Read the model definition and answer for the solid it produces. Units are mm, in the model's axes. A direction names the side the tool comes from. Give positions to 0.01 mm unless a question says otherwise; leave off trailing zeros. Loops run counter-clockwise (first coordinate to the right, second up) from the corner with the lowest first, then second, coordinate; pieces in that order, holes last. Notation, with made-up numbers: (-23.75, 59) -> (30.25, 59) arc R27 ccw to (30.25, 93) -> close; hole circle Ø3 at (70.25, 9). An arc over 180 degrees is marked (long way). Write each question's results on one line, items separated by ' | '. Start each with the question number.
Item 1: Section C-C on y = 6.25 is taken. State how many separate pieces and enclosed holes the cut face has, and give its area (3 significant figures).
Item 2: Section B-B on z = -1.5 is taken. Write down the section's boundary in (x, y).
Item 3: Find the intervals of material crossed by line 1 (Z direction, x = 0, y = 20.25); line 2 (Z direction, x = 0, y = 15.5); line 3 (Z direction, x = 2.25, y = 6.5), in increasing order.
Item 4: Determine the mould class of faces 1 (the flat face through (-2.6, 25.4, 0.2)), 2 (the flat face through (0, 20.32, 0)), 3 (the flat face through (-0.44, 22.9, -1.78)), 4 (the flat face through (3, 13, 12.7)) for opening direction Z: +Z half, -Z half, draft (parallel to the pull), parting line (faces both ways), or undercut.
Item 5: Which of the six approach directions +Z, -Z, +X, -X, +Y, -Y give full straight-line access (tool end or side, diameter ignored) to faces 5 (the flat face through (-4, 23, -0.177)), 6 (the cylindrical face through (-0.69, 12.88, -4.84))?
Item 6: Section A-A on z = -6.75 is taken. Write down the section's boundary in (x, y).
Autodesk Inventor part; units mm, degrees
ref_plane "YZ Plane" through (0, 0, 0) normal (1, 0, 0) x (0, 1, 0)
ref_plane "XZ Plane" through (0, 0, 0) normal (0, 1, 0) x (-1, 0, 0)
ref_plane "XY Plane" through (0, 0, 0) normal (0, 0, 1) x (1, 0, 0)
sketch "Sketch1" plane through (0, 0, 0) normal (0, 1, 0) x (-1, 0, 0)
  line L0 (12.7, 12.7) -> (-12.7, 12.7)
  line L1 (-12.7, 12.7) -> (-12.7, -12.7)
  line L2 (-12.7, -12.7) -> (12.7, -12.7)
  line L3 (12.7, -12.7) -> (12.7, 12.7)
  line L4 (12.7, 12.7) -> (-12.7, -12.7) construction
  line L5 (-12.7, 12.7) -> (12.7, -12.7) construction
  point P0 (0, 0)
  dimension "d0" = 25.4
  dimension "d1" = 25.4
extrude "Extrusion1" add sketch "Sketch1" along normal blind 25.4
sketch "Sketch2" plane through (0, 25.4, 0) normal (0, 1, 0) x (1, 0, 0)
  line L0 (-12.7, 12.7) -> (-12.7, -12.7) construction
  line L1 (-12.7, 0) -> (12.7, 0) construction
  line L2 (12.7, -12.7) -> (12.7, 12.7) construction
  line L3 (-6.1256, -2.4906) -> (-10.5058, -0.671)
  line L4 (-10.5058, -0.671) -> (-10.5058, 0.0782)
  line L5 (-10.5058, 0.0782) -> (-6.1256, 1.8978)
  line L6 (-6.1256, 1.8978) -> (-6.1256, 0.9551)
  line L7 (-6.1256, 0.9551) -> (-9.1885, -0.3005)
  line L8 (-9.1885, -0.3005) -> (-6.1256, -1.5479)
  line L9 (-6.1256, -1.5479) -> (-6.1256, -2.4906)
  line L10 (-2.7705, -0.7698) -> (-5.0306, -0.7698)
  line L11 (-5.0306, -0.7698) -> (-5.0306, 0.177)
  line L12 (-5.0306, 0.177) -> (-2.7705, 0.177)
  line L13 (-2.7705, 0.177) -> (-2.7705, -0.7698)
  line L14 (2.433, -2.54) -> (0.9592, -2.54)
  line L15 (0.9592, -2.54) -> (-0.0206, -0.9221)
  line L16 (-0.0206, -0.9221) -> (-1.0209, -2.54)
  line L17 (-1.0209, -2.54) -> (-2.433, -2.54)
  line L18 (-2.433, -2.54) -> (-0.7822, 0.0165)
  line L19 (-0.7822, 0.0165) -> (-2.3671, 2.54)
  line L20 (-2.3671, 2.54) -> (-0.8933, 2.54)
  line L21 (-0.8933, 2.54) -> (0.0247, 1.0045)
  line L22 (0.0247, 1.0045) -> (0.9674, 2.54)
  line L23 (0.9674, 2.54) -> (2.3794, 2.54)
  line L24 (2.3794, 2.54) -> (0.7863, 0.07)
  line L25 (0.7863, 0.07) -> (2.433, -2.54)
  line L26 (5.1088, -0.7698) -> (2.8488, -0.7698)
  line L27 (2.8488, -0.7698) -> (2.8488, 0.177)
  line L28 (2.8488, 0.177) -> (5.1088, 0.177)
  line L29 (5.1088, 0.177) -> (5.1088, -0.7698)
  line L30 (10.5881, -0.671) -> (6.208, -2.4906)
  line L31 (6.208, -2.4906) -> (6.208, -1.5479)
  line L32 (6.208, -1.5479) -> (9.2667, -0.2964)
  line L33 (9.2667, -0.2964) -> (6.208, 0.9551)
  line L34 (6.208, 0.9551) -> (6.208, 1.8978)
  line L35 (6.208, 1.8978) -> (10.5881, 0.0782)
  line L36 (10.5881, 0.0782) -> (10.5881, -0.671)
  point P0 (0, 0)
extrude "Extrusion2" cut sketch "Sketch2" against normal blind 5.08
sketch "Sketch3" plane through (-12.7, 0, 12.7) normal (0, 0, 1) x (1, 0, 0)
  line L0 (12.6794, 25.4) -> (11.6791, 25.4) construction
  line L1 (12.7, 0) -> (12.6794, 25.4) construction
  line L2 (11.9178, 15.2517) -> (11.916, 17.5118)
  line L3 (11.916, 17.5118) -> (12.8628, 17.5126)
  line L4 (12.8628, 17.5126) -> (12.8647, 15.2525)
  line L5 (12.8647, 15.2525) -> (11.9178, 15.2517)
  line L6 (10.1514, 10.6602) -> (10.1481, 14.6863)
  line L7 (10.1481, 14.6863) -> (11.0991, 14.6871)
  line L8 (11.0991, 14.6871) -> (14.2626, 12.3472)
  line L9 (14.2626, 12.3472) -> (14.2608, 14.5661)
  line L10 (14.2608, 14.5661) -> (15.2282, 14.5669)
  line L11 (15.2282, 14.5669) -> (15.2312, 10.8001)
  line L12 (15.2312, 10.8001) -> (14.2638, 10.7994)
  line L13 (14.2638, 10.7994) -> (11.1168, 13.131)
  line L14 (11.1168, 13.131) -> (11.1188, 10.661)
  line L15 (11.1188, 10.661) -> (10.1514, 10.6602)
  line L16 (11.9238, 7.8911) -> (11.922, 10.1511)
  line L17 (11.922, 10.1511) -> (12.8688, 10.1519)
  line L18 (12.8688, 10.1519) -> (12.8706, 7.8918)
  line L19 (12.8706, 7.8918) -> (11.9238, 7.8911)
extrude "Extrusion3" cut sketch "Sketch3" against normal blind 5.08
sketch "Sketch11" plane through (0, 25.4, 0) normal (0, 1, 0) x (1, 0, 0)
  circle A0 centre (0, 7.9375) radius 3.175
  circle A1 centre (0, -7.9375) radius 3.175
  line L0 (12.7, 12.7) -> (-12.7, 12.7)
  line L1 (-12.7, -12.7) -> (12.7, -12.7)
  point P0 (0, 0)
  dimension "d81" = 6.35
  dimension "d82" = 4.7625
  dimension "d83" = 4.7625
extrude "Extrusion4" cut sketch "Sketch11" against normal blind 25.4
equation "\"d46\" = 0.125 * Sketch7_Pitch"
equation "\"Sketch7_Pitch\" = 1.27"
equation "\"d48\" = 60deg"
equation "\"d67\" = 0.125 * Sketch9_Pitch"
equation "\"Sketch9_Pitch\" = 1.27"
equation "\"d69\" = 60deg"
equation "\"d99\" = 0.125 * Sketch12_Pitch"
equation "\"Sketch12_Pitch\" = 1.27"
equation "\"d101\" = 60deg"
equation "\"d120\" = 0.125 * Sketch14_Pitch"
equation "\"Sketch14_Pitch\" = 1.27"
equation "\"d122\" = 60deg"
equation "\"d143\" = 55deg"
equation "\"Sketch16_Pitch\" = 1.27"
equation "\"d161\" = 55deg"
equation "\"Sketch18_Pitch\" = 1.27"
properties part number "squareCalibrationBlock-1in"
Findings:
1) separate pieces: 1 | enclosed holes: 2 | area: 582 mm2
2) outline: (-12.7, 0) -> (12.7, 0) -> (12.7, 25.4) -> (7.17, 25.4) -> (7.17, 20.32) -> (6.21, 20.32) -> (6.21, 25.4) -> (1.71, 25.4) -> (1.71, 20.32) -> (0.33, 20.32) -> (0.33, 25.4) -> (-0.27, 25.4) -> (-0.27, 20.32) -> (-1.71, 20.32) -> (-1.71, 25.4) -> (-6.13, 25.4) -> (-6.13, 20.32) -> (-7.08, 20.32) -> (-7.08, 25.4) -> (-12.7, 25.4) -> close
3) line 1: -12.7 to -11.11, -4.76 to 4.76, 11.11 to 12.7 | line 2: -12.7 to -11.11, -4.76 to 4.76 | line 3: -12.7 to -10.18, -5.7 to 5.7, 10.18 to 12.7
4) face 1: draft | face 2: undercut | face 3: undercut | face 4: +Z half
5) face 5: +Y | face 6: +Y, -Y
6) outline: (-12.7, 0) -> (-2.94, 0) -> (-2.94, 25.4) -> (-12.7, 25.4) -> close; (2.94, 0) -> (12.7, 0) -> (12.7, 25.4) -> (2.94, 25.4) -> close
